Could you check a few things on this model? Use its own coordinates, in mm. A direction names the side the tool comes from. Coordinates: 2 decimals unless noted, no trailing zeros. Loops run counter-clockwise (first coordinate to the right, second up) from the corner with the lowest first, then second, coordinate; pieces in that order, holes last. Notation, with made-up numbers: (77.25, 15) - (118.25, 15) arc R30 cw to (118.25, 54) - close; hole circle Ø3 at (63.5, 70.25). An arc over 180 degrees is marked (long way). Use CSV: the item, a comma, the result in double quotes.
from build123d import *

# Parameters (mm, degrees)
SKETCH1_W               = 270
SKETCH1_H               = 70
BOSS_EXTRUDE1_DEPTH     = 4
BOSS_EXTRUDE4_DEPTH     = 70
SKETCH7_R               = 3
CUT_EXTRUDE1_DEPTH      = 304.970702227
CUT_EXTRUDE2_DEPTH      = 10
SKETCH9_W               = 4
SKETCH9_H               = 70
BOSS_EXTRUDE5_DEPTH     = 45
SKETCH10_W              = 13
SKETCH10_H              = 4
BOSS_EXTRUDE6_DEPTH     = 43
BOSS_EXTRUDE7_REACH     = 313.858
BOSS_EXTRUDE8_REACH     = 276.704
BOSS_EXTRUDE9_START     = -155.441370069
BOSS_EXTRUDE9_DEPTH     = 24.603121834
SKETCH14_R              = 3
CUT_EXTRUDE3_DEPTH      = 4
CUT_EXTRUDE4_REACH      = 322.045
SKETCH15_W              = 7
SKETCH15_H              = 3.80460454
CUT_EXTRUDE5_DEPTH      = 10
CUT_EXTRUDE5_DEPTH_BACK = 304.645223857
CUT_EXTRUDE6_DEPTH      = 70


# Read off the part's stored shape, not the designer's step: Boss-Extrude9
with BuildPart() as part:
    # Sketch1 → Boss-Extrude1 (new body)
    with BuildSketch(Plane.XY):
        with Locations((135, -35)):
            Rectangle(SKETCH1_W, SKETCH1_H)
    extrude(amount=BOSS_EXTRUDE1_DEPTH)


with BuildPart() as body_2:
    # Mirror1: mirrored copy
    add(part.part.mirror(Plane(origin=(135, 0, 0), x_dir=(0, 0, 1), z_dir=(1, 0, 0))))


with BuildPart() as part_1:
    add(part.part)

    add(body_2.part)  # Boss-Extrude4 merges body 2
    # Sketch2 → Boss-Extrude4 (add, along a direction that is not the sketch's normal)
    with BuildSketch(Plane.XZ.offset(70)):
        Polygon((200.361038291, 14.593997741), (40, 0), (0, 0), (0, 4), (40, 4), (200, 18.561140682), align=None)
    extrude(amount=BOSS_EXTRUDE4_DEPTH, dir=(0, -0.9510565162951534, -0.30901699437494823))

    # Sketch7 → Cut-Extrude1 (cut, through all)
    with BuildSketch(Plane(origin=(0, -15.671129003, 48.230775743), x_dir=(-1, 0, 0), z_dir=(0, 0.3090169943749448, -0.9510565162951545))):
        with Locations((-8, -146.441370146)):
            Circle(SKETCH7_R)
        with Locations(Location((-15, -54.441370146, 0), (0, 0, 270))):
            Circle(SKETCH7_R)
        with Locations(Location((-255, -54.441370146, 0), (0, 0, 270))):
            Circle(SKETCH7_R)
        with Locations((-262, -146.441370146)):
            Circle(SKETCH7_R)
        with Locations(Location((-10, -6.441370146, 0), (0, 0, 270))):
            Circle(SKETCH7_R)
        with Locations(Location((-260, -6.441370146, 0), (0, 0, 270))):
            Circle(SKETCH7_R)
    extrude(amount=CUT_EXTRUDE1_DEPTH, mode=Mode.SUBTRACT)

    # Sketch8 → Cut-Extrude2 (cut)
    with BuildSketch(Plane(origin=(0, 0, 0), x_dir=(-1, 0, 0), z_dir=(0, 0, -1))):
        with BuildLine():
            Line((-270, -70), (-270, -21))
            Line((-270, -21), (-240, -21))
            ThreePointArc((-240, -21), (-205.351767722, -35.351767722), (-191, -70))
            Line((-191, -70), (-270, -70))
        make_face()
    extrude(amount=-CUT_EXTRUDE2_DEPTH, mode=Mode.SUBTRACT)

    # Sketch9 → Boss-Extrude5 (add)
    with BuildSketch(Plane(origin=(0, 0, 0), x_dir=(-1, 0, 0), z_dir=(0, 0, -1))):
        Polygon((-243, 0), (-155, -70), (-148.574540436, -70), (-152.509905737, -66.869595783), (-236.574540436, 0), align=None)
        with Locations((-25, -35)):
            Rectangle(SKETCH9_W, SKETCH9_H)
    extrude(amount=BOSS_EXTRUDE5_DEPTH)

    # Sketch10 → Boss-Extrude6 (add)
    with BuildSketch(Plane(origin=(0, -6.684405197, 20.57248383), x_dir=(-1, 0, 0), z_dir=(0, 0.3090169943749482, -0.9510565162951534))):
        with Locations((-33.5, -134.573956141)):
            Rectangle(SKETCH10_W, SKETCH10_H)
        Polygon((-23, -66.573956141), (-27, -66.573956141), (-27, -132.573956141), (-27, -136.573956141), (-23, -136.573956141), align=None)
    extrude(amount=BOSS_EXTRUDE6_DEPTH)

    # Boss-Extrude7: up to this plane
    boss_extrude7_end = Plane(origin=(0, 6.603325561, -20.32294637), z_dir=(0, 0.30901699437494823, -0.9510565162951534))
    # Sketch11 → Boss-Extrude7 (add, up to the surface)
    with BuildSketch(Plane(origin=(-1.560893066, -5.572804076, 17.151327361), x_dir=(-0.9962752106554099, 0.026646699794247903, -0.08201010927680777), z_dir=(0.08623053191021567, 0.30786597116700337, -0.947514031117154)), mode=Mode.PRIVATE) as boss_extrude7_sk1:
        Polygon((-41.716277412, -132.573956141), (-202.676859965, -128.064162823), (-202.676859965, -132.064162823), (-41.716277412, -136.573956141), align=None)
    boss_extrude7_tool1 = split(extrude(boss_extrude7_sk1.sketch, amount=BOSS_EXTRUDE7_REACH, mode=Mode.PRIVATE), bisect_by=boss_extrude7_end, keep=Keep.BOTH, mode=Mode.PRIVATE)
    add(boss_extrude7_tool1.solids().sort_by_distance((120.180519, -134.671843, -13.716157))[0])

    # Boss-Extrude8: up to this face of the body (flat: up to its plane)
    boss_extrude8_end = Plane(part_1.part.faces().sort_by_distance((41.860887851, -128.027977729, -41.460870718))[0])
    # Sketch12 → Boss-Extrude8 (add, up to the picked face)
    with BuildSketch(Plane(origin=(40, 0, 0), x_dir=(0, 0, -1), z_dir=(1, 0, 0)), mode=Mode.PRIVATE) as boss_extrude8_sk1:
        Polygon((20.395121629, -132.769730075), (21.631189606, -136.573956141), (62.526619807, -123.286225383), (61.290551829, -119.481999317), align=None)
    boss_extrude8_tool1 = split(extrude(boss_extrude8_sk1.sketch, amount=BOSS_EXTRUDE8_REACH, mode=Mode.PRIVATE), bisect_by=boss_extrude8_end, keep=Keep.BOTH, mode=Mode.PRIVATE)
    add(boss_extrude8_tool1.solids().sort_by(Axis((40, -128.027978, -41.460871), (1, 0, 0)))[0])

    # Boss-Extrude9 outline → Boss-Extrude9 (add)
    with BuildSketch(Plane(origin=(0, 0, 0), x_dir=(1, 0, 0), z_dir=(0, 0.9510565162951545, 0.3090169943749449)).offset(BOSS_EXTRUDE9_START)):
        Polygon((200.361038291, -35.510906256), (40, -21.631189606), (0, -21.631189606), (0, -25.435415671), (40, -25.435415671), (200, -39.283883402), align=None)
    extrude(amount=BOSS_EXTRUDE9_DEPTH)

    # Sketch14 → Cut-Extrude3 (cut)
    with BuildSketch(Plane(origin=(0, -6.684405197, 20.57248383), x_dir=(-1, 0, 0), z_dir=(0, 0.3090169943749481, -0.9510565162951534))):
        with Locations(Location((-8, -146.441370069, 0), (0, 0, 90))):
            Circle(SKETCH14_R)
    extrude(amount=-CUT_EXTRUDE3_DEPTH, mode=Mode.SUBTRACT)

    # Cut-Extrude4: up to this plane
    cut_extrude4_end = Plane(origin=(200.361038291, -136.573956141, -7.037191865), z_dir=(0.08623053191021565, 0.3078659711670031, -0.9475140311171542))
    # Sketch15 → Cut-Extrude4 (cut, up to the surface)
    with BuildSketch(Plane(origin=(0, 6.603325561, -20.32294637), x_dir=(-1, 0, 0), z_dir=(0, 0.3090169943749483, -0.9510565162951534)), mode=Mode.PRIVATE) as cut_extrude4_sk1:
        with Locations((-201.784144044, -130.161860553)):
            Rectangle(SKETCH15_W, SKETCH15_H)
    cut_extrude4_tool1 = split(extrude(cut_extrude4_sk1.sketch, amount=-CUT_EXTRUDE4_REACH, mode=Mode.PRIVATE), bisect_by=cut_extrude4_end, keep=Keep.BOTH, mode=Mode.PRIVATE)
    add(cut_extrude4_tool1.solids().sort_by_distance((201.784144, -117.18796, -60.545173))[0], mode=Mode.SUBTRACT)

    # Sketch16 → Cut-Extrude5 (cut, two sides: drawn at the far end of the back side and taken through both)
    with BuildSketch(Plane(origin=(0, -125.600482622, -40.81007066), x_dir=(1, 0, 0), z_dir=(0, 0.9510565162951534, 0.3090169943749483)).offset(-CUT_EXTRUDE5_DEPTH_BACK)):
        Polygon((205.284144044, 21.368810394), (198.284144044, 21.368810394), (198.284144044, -35.331144988), (200.361038291, -35.510906256), align=None)
    extrude(amount=CUT_EXTRUDE5_DEPTH + CUT_EXTRUDE5_DEPTH_BACK, mode=Mode.SUBTRACT)

    # Sketch17 → Cut-Extrude6 (cut)
    with BuildSketch(Plane(origin=(243, 0, 0), x_dir=(0, 0, -1), z_dir=(1, 0, 0))):
        Polygon((-13.772265004, -28.596864407), (35.94568304, -12.442523831), (38.417818995, -20.050975962), (-11.300129049, -36.205316538), align=None)
    extrude(amount=-CUT_EXTRUDE6_DEPTH, mode=Mode.SUBTRACT)


solid = part_1.part
(1) Suppose I cut it at A-A (x = 106.5). Write out the boundary of the cut face in (y, z), plus the area to 3 significant figures.
Computed:
outline,"(-157.47, -18.37) - (-156.3, -21.99) - (-136.57, -15.58) - (-121.62, -61.99) - (-117.82, -60.75) - (-132.77, -14.34) - (-70, 6.05) - (-70, 10.05) - close; (-70, 0) - (0, 0) - (0, 4) - (-70, 4) - close"
area,"823 mm²"
(2) Thinking about a two-plate mould opening in X: for faces 1 (the face through (149, -70, -12)), 2 (the face through (27, -61, -23)), 3 (the face through (23, -65, -24)), which applies, +X half, -X half, draft (parallel to the pull), parting line (faces both ways), or undercut?
Computed:
face 1,"draft"
face 2,"undercut"
face 3,"-X half"
(3) Will these pins go through, and if not, where does the flat tip stop? pin 1 (4.5 mm diameter, centred on x = 248.5, z = 2, fed in from -Y); pin 2 (1 mm diameter, centred on y = -74, z = -11, fed in from +X); pin 3 (11 mm diameter, centred on x = 185.5, y = -45, fed in from -Z).
Computed:
pin 1,"stops at y = -21"
pin 2,"stops at x = 27"
pin 3,"stops at z = -45"
(4) Which directions (+Z, -Z, +X, -X, +Y, -Y) give clear straight access to the entire face, cutting with the end or side of a thin tool? Please do faces 4 (the face through (199.616, -34.51, -22.185)), 5 (the face through (195.695, -49.071, 1.972)), 6 (the face through (11, -35, 0)).
Computed:
face 4,"-Z, +X"
face 5,"+Z, -Z, +X"
face 6,"-Z, -X, +Y"
(5) Please list where these lines run through material, in increasing order: line 1 (Y direction, x = 184, z = -34) (3 decimals); line 2 (Y direction, x = 156, z = -42); line 3 (Z direction, x = 108, y = -63).
Computed:
line 1,"y = -128.365 to -124.162, -46.932 to -41.821"
line 2,"y = -126.61 to -122.41, -69.2 to -64.09"
line 3,"z = 0 to 4"
(6) Suppose I cut it at C-C (x = 248). Write out the boundary of the cut face in (y, z), plus the area to 3 significant figures.
Computed:
outline,"(-21, 0) - (0, 0) - (0, 4) - (-21, 4) - close"
area,"84.0 mm²"
(7) Suppose I cut it at D-D (x = 69.5). Write out the boundary of the cut face in (y, z), plus the area to 3 significant figures.
Computed:
outline,"(-156.48, -21.42) - (-155.31, -25.03) - (-136.57, -18.95) - (-122.6, -62.3) - (-118.8, -61.07) - (-132.77, -17.71) - (-70, 2.68) - (-70, 0) - (0, 0) - (0, 4) - (-70, 4) - (-70, 6.68) - close"
area,"806 mm²"
(8) Suppose I cut it at B-B (z = -57). Write out the boundary of the cut face in (x, y).
Computed:
outline,"(23, -125.08) - (43.22, -125.08) - (198.28, -120.53) - (198.28, -116.33) - (43.33, -120.88) - (27, -120.88) - (27, -106.28) - (23, -106.28) - close"
